Work out the finished part from the listing and answer in its coordinate system (mm). Give positions to 0.01 mm unless a question says otherwise; leave off trailing zeros. Loops run counter-clockwise (first coordinate to the right, second up) from the corner with the lowest first, then second, coordinate; pieces in that order, holes last. Notation, with made-up numbers: (-19.5, -18) - (2.5, -18) arc R21 cw to (2.5, 4) - close; hole circle Ø3 at (-20.75, 28.5). An arc over 180 degrees is marked (long way). One line per item, written item: value.
from build123d import *

# Parameters (mm, degrees)
F0_R     = 14.15
F0_R_2   = 9.0475
F1_DEPTH = 1.65
F2_SIZE  = 1
F3_R     = 1.2


with BuildPart() as f1:
    # F0 (on Top) → F1 (new body)
    with BuildSketch(Plane.XY):
        Circle(F0_R)
        Circle(F0_R_2, mode=Mode.SUBTRACT)
    extrude(amount=F1_DEPTH)

    # F2
    f2_edges = [f1.edges().sort_by_distance(p)[0] for p in [
        (-14.15, 0, 0),
    ]]
    chamfer(f2_edges, length=F2_SIZE)

    # F3
    f3_edges = [f1.edges().sort_by_distance(p)[0] for p in [
        (-13.15, 0, 0),
    ]]
    fillet(f3_edges, radius=F3_R)


solid = f1.part
1. The mould has two halves that part along X. Classify faces 1 (the cylindrical face through (-7.18, -5.505, 0.813)), 2 (the flat face through (-9, 3, 0)), 3 (the cylindrical face through (6.529, -12.553, 1.32)): released by +X, released by -X, zero draft, split by the parting line, or undercut.
Output:
face 1: undercut
face 2: zero draft
face 3: split by the parting line
2. Find the intervals of material crossed by line 1 along Y through (x, z) = (0, 1.1); line 2 along Y through (x, z) = (0, 0.35); line 3 along X through (y, z) = (3.25, 1.05), in increasing order.
Output:
line 1: y = -14.15 to -9.05, 9.05 to 14.15
line 2: y = -13.5 to -9.05, 9.05 to 13.5
line 3: x = -13.77 to -8.44, 8.44 to 13.77
3. Section C-C (z = 0.75) is taken. Write down the section's boundary in (x, y) (1 decimal), and give its area (3 significant figures).
Output:
outline: circle Ø27.8 at (0, 0); hole circle Ø18.1 at (0, 0)
area: 350 mm²
4. Section A-A (x = 0) is taken. Write down the section's boundary in (y, z).
Output:
outline: (-14.15, 1) - (-13.5, 0.35) arc R1.2 ccw to (-12.65, 0) - (-9.05, 0) - (-9.05, 1.65) - (-14.15, 1.65) - close; (9.05, 0) - (12.65, 0) arc R1.2 ccw to (13.5, 0.35) - (14.15, 1) - (14.15, 1.65) - (9.05, 1.65) - close
